Source: three-view drawing plus pictorial views. Frame: mm from the lowest corner of the part. A direction names the side the tool comes from. Coordinates: 2 decimals unless noted, no trailing zeros. Loops run counter-clockwise (first coordinate to the right, second up) from the corner with the lowest first, then second, coordinate; pieces in that order, holes last. Notation, with made-up numbers: M 27.5,-19 L 51.5,-19 A24 cw 51.5,19 Z; hole C 82.5,78 d6. An arc over 180 degrees is marked long. Use a Markdown table: item, result. Add a question column.
1. Pin query (flat end, axial travel): pin 1 (10 mm diameter, centred on x = 56, y = 17.5, fed in from -Z). Return the tip coordinate at first contact, or that it passes through.
2. Section A-A on x = 26. Output: boundary loops of the cut face in (y, z) (1 decimal).
3. Line query: L1, parallel to X at y = 36, z = 13.75 (1 decimal). Output: solid intervals per line, ascending. Write a range as [from, to].
4. Set-up query: the marked faces 4 and 5. Return all of +Z, -Z, +X, -X, +Y, -Y with unobstructed straight access to the full face (end or side cutting, diameter ignored); none if empty.
5. Draft query along Y for the marked faces 1, 2 and 3. Return one class per face: +Y half, -Y half, draft (parallel to the pull), parting line (faces both ways), or undercut.
6. Section C-C on z = 7.75. Output: boundary loops of the cut face in (x, y) (1 decimal).
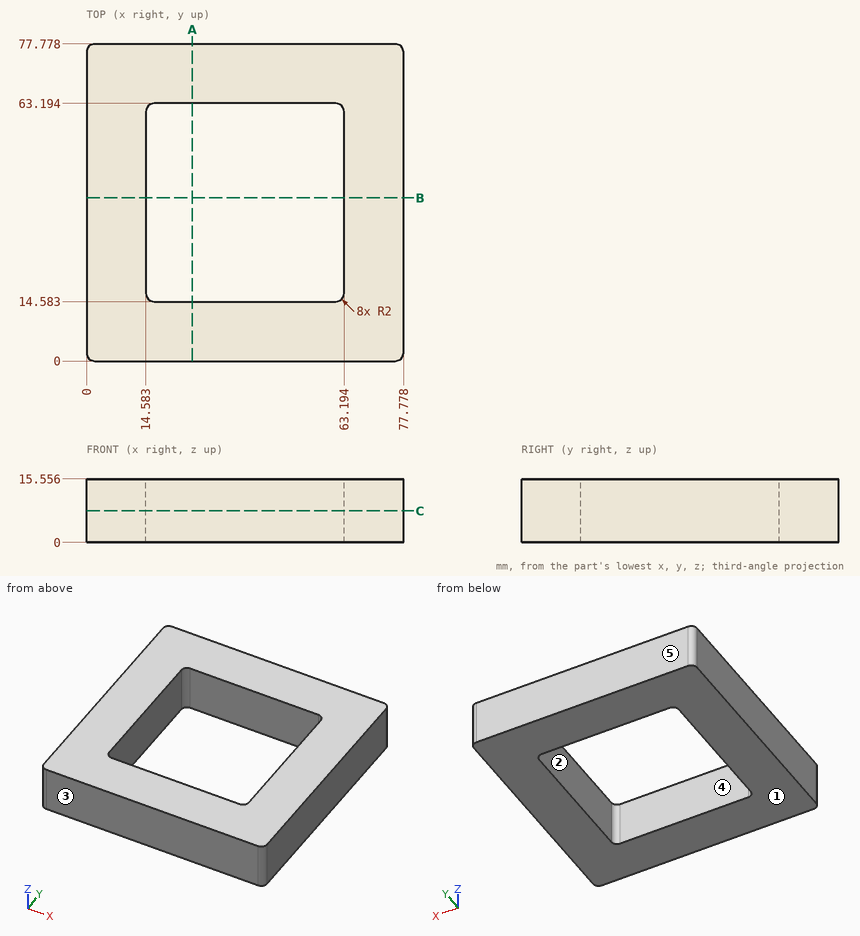
Answers below:
| question | item | result |
|---|---|---|
| 1 | pin 1 | stops at z = 0 |
| 2 | outline | M 0,0 L 14.6,0 L 14.6,15.6 L 0,15.6 Z; M 63.2,0 L 77.8,0 L 77.8,15.6 L 63.2,15.6 Z |
| 3 | L1 | x = [0, 14.6], [63.2, 77.8] |
| 4 | face 4 | +Z, -Z |
| 4 | face 5 | +Z, -Z, +X, -X, +Y |
| 5 | face 1 | draft |
| 5 | face 2 | undercut |
| 5 | face 3 | -Y half |
| 6 | outline | M 0,2 A2 ccw 2,0 L 75.8,0 A2 ccw 77.8,2 L 77.8,75.8 A2 ccw 75.8,77.8 L 2,77.8 A2 ccw 0,75.8 Z; hole M 14.6,16.6 A2 ccw 16.6,14.6 L 61.2,14.6 A2 ccw 63.2,16.6 L 63.2,61.2 A2 ccw 61.2,63.2 L 16.6,63.2 A2 ccw 14.6,61.2 Z |
